from build123d import *

# Parameters (mm, degrees)
SKETCH_W        = 48
SKETCH_H        = 75
PAD_DEPTH       = 1.5
FILLET014_R     = 3
FILLET015_R     = 3
FILLET016_R     = 3
FILLET017_R     = 3
SKETCH016_R     = 1.6
POCKET012_DEPTH = 1.501


with BuildPart() as part:
    # Sketch → Pad (new body)
    with BuildSketch(Plane.XY):
        with Locations((-5, 0)):
            Rectangle(SKETCH_W, SKETCH_H)
    extrude(amount=PAD_DEPTH)

    # Fillet014
    fillet014_edges = [part.edges().sort_by_distance(p)[0] for p in [
        (19, 37.5, 0.75),
    ]]
    fillet(fillet014_edges, radius=FILLET014_R)

    # Fillet015
    fillet015_edges = [part.edges().sort_by_distance(p)[0] for p in [
        (-29, 37.5, 0.75),
    ]]
    fillet(fillet015_edges, radius=FILLET015_R)

    # Fillet016
    fillet016_edges = [part.edges().sort_by_distance(p)[0] for p in [
        (-29, -37.5, 0.75),
    ]]
    fillet(fillet016_edges, radius=FILLET016_R)

    # Fillet017
    fillet017_edges = [part.edges().sort_by_distance(p)[0] for p in [
        (19, -37.5, 0.75),
    ]]
    fillet(fillet017_edges, radius=FILLET017_R)

    # Sketch016 → Pocket012 (cut, through all)
    with BuildSketch(Plane(origin=(0, 0, 0), x_dir=(1, 0, 0), z_dir=(0, 0, -1))):
        with Locations((-8.35928, 33.2899)):
            Circle(SKETCH016_R)
        with Locations((8.35928, 33.2899)):
            Circle(SKETCH016_R)
    extrude(amount=-POCKET012_DEPTH, mode=Mode.SUBTRACT)


solid = part.part
Build history of the part. All positions in model axes, mm. Round coordinates to 2 decimals unless told otherwise and drop trailing zeros. Loops run counter-clockwise (first coordinate to the right, second up) from the corner with the lowest first, then second, coordinate; pieces in that order, holes last. Notation, with made-up numbers: (-22, 57) -> (34, 57) arc R16 ccw to (34, 77) -> close; hole circle Ø7 at (-6, -26). An arc over 180 degrees is marked (long way). Use CSV: the item, a comma, the result in double quotes. Start each with the question number.
Q1. Flat gauge pin, fed straight in: pin 1 Ø1.9 at (x, y) = (-8.36, -33.29) entering from -Z. Where does the tip first touch, or does it go through?
Q2. Saw through at A-A on x = 9. Give the cut face in (y, z), and give its area (3 significant figures).
Q3. Drill centre lines: L1, parallel to X at y = -33.5, z = 0.9; L2, parallel to Y at x = -8, z = 0.75. Where is each one in solid material? Low to high.
Q4. Mould opens along Y. For faces 1 (the face through (8.01, -31.73, 0.74)), 2 (the face through (-5, 37.5, 1)), 3 (the face through (-28.14, -36.6, 0.76)) say: +Y half, -Y half, draft (parallel to the pull), parting line (faces both ways), or undercut.
Solutions:
1,pin 1,"passes through"
2,outline,"(-37.5, 0) -> (-34.76, 0) -> (-34.76, 1.5) -> (-37.5, 1.5) -> close; (-31.82, 0) -> (37.5, 0) -> (37.5, 1.5) -> (-31.82, 1.5) -> close"
2,area,"108 mm^2"
3,L1,"x = -29 to -9.95, -6.77 to 6.77, 9.95 to 19"
3,L2,"y = -37.5 to -34.85, -31.73 to 37.5"
4,face 1,"undercut"
4,face 2,"+Y half"
4,face 3,"-Y half"
